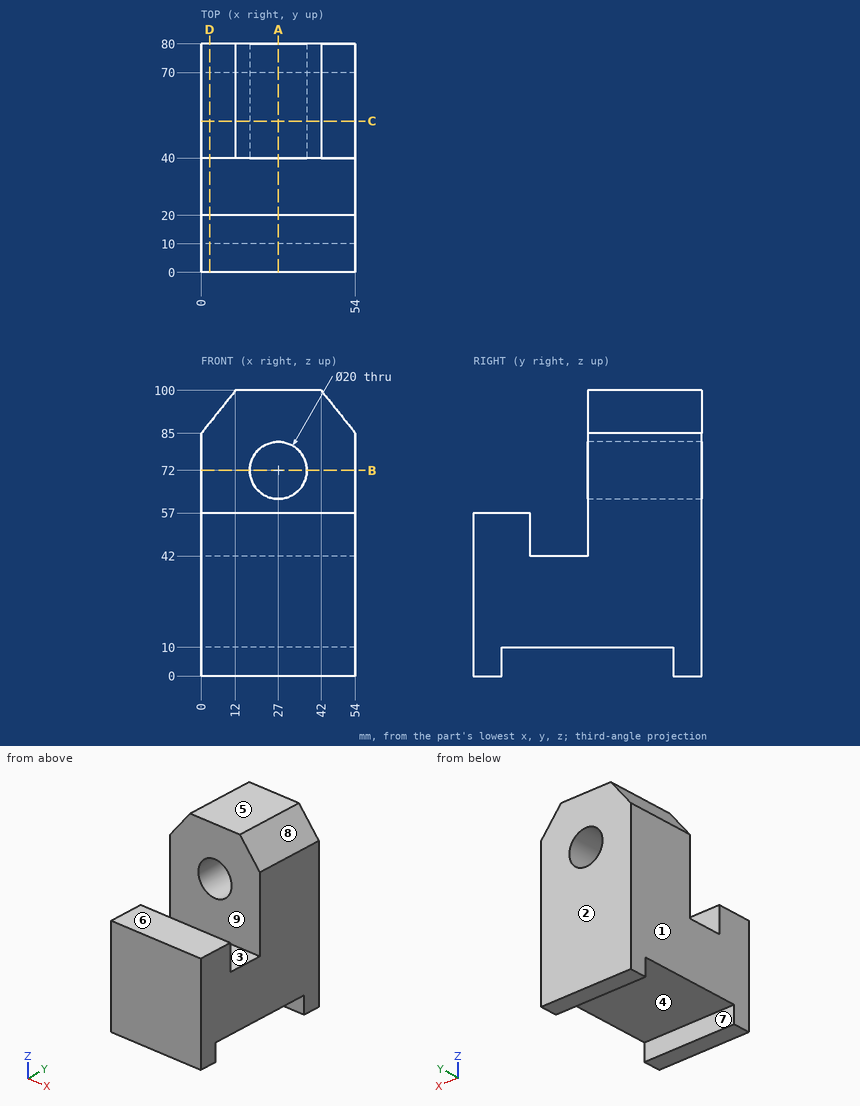
The drawing under review shows one solid part. Ordinate dimensions are in mm from its lowest x, y, z. A direction names the side the tool comes from. Coordinates: 2 decimals unless noted, no trailing zeros. Write each loop counter-clockwise with the first axis right and the second up, starting at its lowest first coordinate (ties: lowest second). Pieces come first, ordered by that corner, then holes. Notation, with made-up numbers: (58, 85.25) -> (111, 85.25) arc R9 cw to (111, 101.25) -> close; hole circle Ø11 at (84, 79). An arc over 180 degrees is marked (long way). One line per item, written item: value. Start each with the question number.
Q1. Clearance check with flat-ended pins moving along their axes: P1, Ø8, axis at x = 24.5, z = 5.5, coming from the -Y side; P2, Ø22, axis at x = 16, y = 7.5, coming from the +Z side; P3, Ø6, axis at x = 47, y = 66, coming from the -Z side; P4, Ø12, axis at x = 40, z = 82.5, coming from the -Y side. State where each tip first meets the part, or that it passes through.
Q2. Add section D-D, the plane x = 3. Give the boundary of the cut face in (y, z).
Q3. For the marked faces 5, 6, 7, 8 and 9, list the 3-axis set-ups (+Z, -Z, +X, -X, +Y, -Y) from which the entire face can be reached by the end or side of a thin tool; tool diameter is ignored.
Q4. Add section B-B, the plane z = 72. Give the boundary of the cut face in (x, y), then the cut area to 3 significant figures.
Q5. Add section C-C, the plane y = 53. Give the boundary of the cut face in (x, z), then the cut area to 3 significant figures.
Q6. To check wall thickness, follow probe 1 along X at (y, z) = (57, 72); probe 2 along Y at (x, z) = (10.5, 42.5); probe 3 along Y at (x, z) = (6.5, 70.5). State the ranges of each line that lie inside material, in increasing order.
Q7. The part is to be moulded in two halves that separate along Y. For the marked faces 1, 2, 3 and 4, say which applies: +Y half, -Y half, draft (parallel to the pull), parting line (faces both ways), or undercut.
Q8. Add section A-A, the plane x = 27. Give the boundary of the cut face in (y, z).
Response:
1. P1: y = 0
1. P2: z = 57
1. P3: z = 10
1. P4: y = 40
2. outline: (0, 0) -> (10, 0) -> (10, 10) -> (70, 10) -> (70, 0) -> (80, 0) -> (80, 88.75) -> (40, 88.75) -> (40, 42) -> (20, 42) -> (20, 57) -> (0, 57) -> close
3. face 5: +Z, +X, -X, +Y, -Y
3. face 6: +Z, +X, -X, -Y
3. face 7: -Z, +X, -X
3. face 8: +Z, +X, +Y, -Y
3. face 9: +Z, +X, -X
4. outline: (0, 40) -> (17, 40) -> (17, 80) -> (0, 80) -> close; (37, 40) -> (54, 40) -> (54, 80) -> (37, 80) -> close
4. area: 1,360 mm²
5. outline: (0, 10) -> (54, 10) -> (54, 85) -> (42, 100) -> (12, 100) -> (0, 85) -> close; hole circle Ø20 at (27, 72)
5. area: 4,370 mm²
6. probe 1: 0 to 17, 37 to 54
6. probe 2: 0 to 20, 40 to 80
6. probe 3: 40 to 80
7. face 1: draft
7. face 2: +Y half
7. face 3: undercut
7. face 4: undercut
8. outline: (0, 0) -> (10, 0) -> (10, 10) -> (70, 10) -> (70, 0) -> (80, 0) -> (80, 62) -> (40, 62) -> (40, 42) -> (20, 42) -> (20, 57) -> (0, 57) -> close; (40, 82) -> (80, 82) -> (80, 100) -> (40, 100) -> close
